Geometry check sheet. Reference: the model listing, model coordinates, mm. Coordinates: 2 decimals unless noted, no trailing zeros. Order: outer loops, then holes, each group sorted by start corner. A loop starts at its lowest first (then second) coordinate and runs counter-clockwise, first axis right, second up. Notation, with made-up numbers: (21.5, -11) - (56.5, -11) arc R10 cw to (56.5, -3) - close; hole circle Ø7 at (17.5, 84.5). An arc over 180 degrees is marked (long way). Put each result on its own line as item: value.
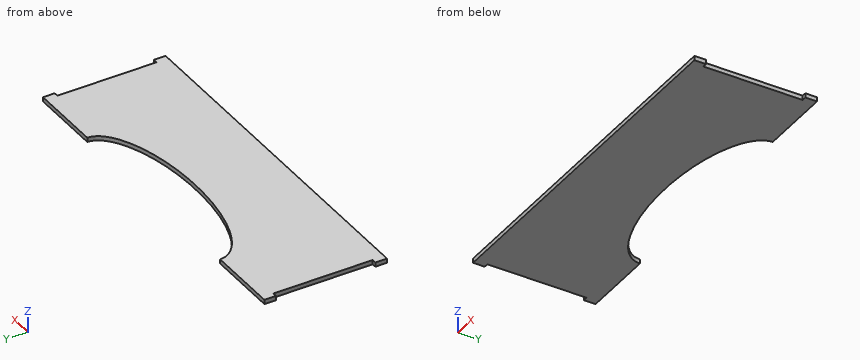
Autodesk Inventor part; units mm, degrees
ref_plane "YZ Plane" through (0, 0, 0) normal (1, 0, 0) x (0, 1, 0)
ref_plane "XZ Plane" through (0, 0, 0) normal (0, 1, 0) x (-1, 0, 0)
ref_plane "XY Plane" through (0, 0, 0) normal (0, 0, 1) x (1, 0, 0)
sketch "Эскиз1" plane through (0, 0, 0) normal (0, 0, 1) x (1, 0, 0)
  line L0 (127.4522, 43.2469) -> (127.4522, -40.7531)
  line L1 (127.4522, -40.7531) -> (-122.5478, -40.7531)
  line L2 (-122.5478, -40.7531) -> (-122.5478, 43.2469)
  line L3 (-119.5478, -40.7531) -> (-122.5478, -40.7531)
  line L4 (-119.5478, 35.2469) -> (-122.5478, 35.2469)
  line L5 (-119.5478, -40.7531) -> (-119.5478, -32.7531)
  line L6 (-122.5478, 35.2469) -> (-119.5478, 35.2469)
  line L7 (-119.5478, 35.2469) -> (-119.5478, -32.7531)
  line L8 (-119.5478, -32.7531) -> (-122.5478, -32.7531)
  line L9 (-122.5478, -32.7531) -> (-122.5478, 35.2469)
  ellipse E0 centre (2.4522, 43.2469) end of major axis (77.4522, 43.2469) minor radius 28.3094 (-72.5478, 43.2469) -> (77.4522, 43.2469) ccw
  line L10 (-122.5478, 43.2469) -> (-72.5478, 43.2469)
  line L11 (77.4522, 43.2469) -> (127.4522, 43.2469)
  line L12 (127.4522, 35.2469) -> (124.4522, 35.2469)
  line L13 (124.4522, 35.2469) -> (124.4522, -32.7531)
  line L14 (124.4522, -32.7531) -> (127.4522, -32.7531)
  line L15 (127.4522, -32.7531) -> (127.4522, 35.2469)
  point P0 (0, 0)
  point P1 (125.9522, -32.7531)
  dimension "d1" = 75
  dimension "d0" = 250
  dimension "d2" = 125
  dimension "d3" = 84
  dimension "d4" = 150
  dimension "d5" = 84
  dimension "d6" = 3
  dimension "d7" = 8
extrude "Выдавливание1" add sketch "Эскиз1" along normal blind 3 contours L0 L12 L13 L14 L1 L5 L7 L4 L2 L10 E0 L11 | L1 L2 L8 L5
properties part number "боковая стенка"
Q1. Section check A-A on y = 0. Record the boundary of the cut face in (x, z), then the cut area to 3 significant figures.
Answer block:
outline: (-119.55, 0) - (124.45, 0) - (124.45, 3) - (-119.55, 3) - close
area: 732 mm^2
Q2. Depth check by flat-ended pin: pin 1 Ø1.5 at (y, z) = (-4.5, 1.5) entering from +X; pin 2 Ø0.9 at (y, z) = (-14.5, 2) entering from -X; pin 3 Ø5 at (x, y) = (23.5, -6) entering from -Z. Enter the tip coordinate at first touch or a pass-through.
Answer block:
pin 1: stops at x = 124.45
pin 2: stops at x = -119.55
pin 3: stops at z = 0
Q3. Thickness scan on L1, parallel to X at y = 10, z = 1.25; L2, parallel to X at y = 24.5, z = 0.45; L3, parallel to X at y = 37.5, z = 2.2. Record the ranges inside material, lowest first. Write a range as [from, to].
Answer block:
L1: x = [-119.55, 124.45]
L2: x = [-119.55, -53.75], [58.65, 124.45]
L3: x = [-122.55, -70.99], [75.89, 127.45]
